Build history of the part. All positions in model axes, mm. A direction names the side the tool comes from. Give positions to 0.01 mm unless a question says otherwise; leave off trailing zeros. Write each loop counter-clockwise with the first axis right and the second up, starting at its lowest first coordinate (ties: lowest second). Pieces come first, ordered by that corner, then holes. Notation, with made-up numbers: M -4,22 L 38,22 A29 ccw 38,47 Z; hole C 4,63 d3. An arc over 180 degrees is marked long. One line per item, written item: value. Start each with the question number.
from build123d import *

# Parameters (mm, degrees)
F1_DEPTH = 40
F2_R     = 3
F3_W     = 40
F3_H     = 40
F3_R     = 7.5
F4_DEPTH = 10


with BuildPart() as f1:
    # F0 (on Top) → F1 (new body)
    with BuildSketch(Plane.XY):
        Polygon((-250, -20), (250, -20), (250, 20), (20, 20), (20, 60), (-20, 60), (-20, 20), (-250, 20), align=None)
    extrude(amount=F1_DEPTH)

    # F2
    f2_edges = [f1.edges().sort_by_distance(p)[0] for p in [
        (250, 20, 20),
        (-250, -20, 20),
        (250, -20, 20),
        (0, -20, 0),
        (0, -20, 40),
        (135, 20, 40),
        (250, 0, 0),
        (250, 0, 40),
        (-250, 0, 40),
        (20, 20, 20),
        (-250, 20, 20),
        (135, 20, 0),
        (-250, 0, 0),
        (20, 40, 0),
        (-20, 40, 40),
        (-135, 20, 40),
        (20, 40, 40),
        (20, 60, 20),
        (0, 60, 40),
        (-135, 20, 0),
        (-20, 20, 20),
        (-20, 60, 20),
        (-20, 40, 0),
        (0, 60, 0),
    ]]
    fillet(f2_edges, radius=F2_R)

    # F3 (on face) → F4 (join)
    with BuildSketch(Plane.XY.offset(40)):
        with Locations((-230, 0)):
            Rectangle(F3_W, F3_H)
        with Locations((-230, 0)):
            Circle(F3_R, mode=Mode.SUBTRACT)
        with Locations((230, 0)):
            Rectangle(F3_W, F3_H)
        with Locations((230, 0)):
            Circle(F3_R, mode=Mode.SUBTRACT)
    extrude(amount=F4_DEPTH)


solid = f1.part
1) Drop flat-ended pins along their axis: P1, Ø8, axis at x = -237, z = 44, coming from the +Y side; P2, Ø8, axis at x = 7.5, y = 24.5, coming from the +Z side; P3, Ø1.5, axis at y = 41, z = 22, coming from the +X side. Give the stop position or say it passes through.
2) Band-saw the part on C-C (z = 32.5). List the corners of the cut face in (x, y), then the cut area to 3 significant figures.
3) Band-saw the part on D-D (x = 230). List the corners of the cut face in (y, z), then the cut area to 3 significant figures.
4) Tool access for faces 1 (the face through (-133, 20, 20)), 2 (the face through (137, 20, 20)), 3 (the face through (230, 0, 40)), 4 (the face through (210, 0, 45)): list every direction of +Z, -Z, +X, -X, +Y, -Y with a clear straight run to the whole face (end or side of a thin tool).
5) Mould opens along X. For faces 5 (the face through (-250, 0, 45)), 6 (the face through (-237.493, 0.33, 44.93)), 7 (the face through (250, 0, 45)) say: released by +X, released by -X, zero draft, split by the parting line, or undercut.
6) Probe line 1 along Y through (x, z) = (-230, 47.25); line 2 along X through (y, z) = (-15, 45.5); line 3 along Y through (x, z) = (167, 18.5). List the from-to ranges inside material, lowest first. Write a range as from..to.
7) Band-saw the part on A-A (x = 55). List the corners of the cut face in (y, z).
Model answer:
1. P1: stops at y = 20
1. P2: stops at z = 40
1. P3: stops at x = 20
2. outline: M -250,-17 A3 ccw -247,-20 L 247,-20 A3 ccw 250,-17 L 250,17 A3 ccw 247,20 L 23,20 A3 cw 20,23 L 20,57 A3 ccw 17,60 L -17,60 A3 ccw -20,57 L -20,23 A3 cw -23,20 L -247,20 A3 ccw -250,17 Z
2. area: 21,600 mm²
3. outline: M -20,3 A3 ccw -17,0 L 17,0 A3 ccw 20,3 L 20,37 A3 ccw 17,40 L 20,40 L 20,50 L 7.5,50 L 7.5,40 L -7.5,40 L -7.5,50 L -20,50 L -20,40 L -17,40 A3 ccw -20,37 Z
3. area: 1,840 mm²
4. face 1: +Z, -Z, -X, +Y
4. face 2: +Z, -Z, +X, +Y
4. face 3: +Z
4. face 4: +Z, +Y, -Y
5. face 5: released by -X
5. face 6: undercut
5. face 7: released by +X
6. line 1: y = -20..-7.5, 7.5..20
6. line 2: x = -250..-210, 210..250
6. line 3: y = -20..20
7. outline: M -20,3 A3 ccw -17,0 L 17,0 A3 ccw 20,3 L 20,37 A3 ccw 17,40 L -17,40 A3 ccw -20,37 Z
